Autodesk Inventor part; units mm, degrees
ref_plane "Work Plane1" through (0, 10, 0) normal (0, 1, 0) x (-1, 0, 0)
ref_plane "YZ Plane" through (0, 0, 0) normal (1, 0, 0) x (0, 1, 0)
ref_plane "XY Plane" through (0, 0, 0) normal (0, 0, 1) x (1, 0, 0)
sketch "Sketch1" plane through (0, 0, 0) normal (0, 1, 0) x (-1, 0, 0)
  circle A0 centre (0, 0) radius 50
  dimension "d0" = 100
extrude "Extrusion1" add sketch "Sketch1" along normal blind 20
sketch "Sketch2" plane through (0, 20, 0) normal (0, 1, 0) x (1, 0, 0)
  line L0 (60.9024, 0) -> (39.0976, 0) construction
  circle A0 centre (0, 0) radius 50
  line L1 (60.9024, 10.5) -> (39.0976, 10.5)
  line L2 (39.0976, -10.5) -> (60.9024, -10.5)
  arc A1 (60.9024, -10.5) -> (60.9024, 10.5) centre (60.9024, 0) ccw
  arc A2 (39.0976, 10.5) -> (39.0976, -10.5) centre (39.0976, 0) ccw
  point P0 (50, 0)
  dimension "d3" = 21
extrude "Extrusion2" cut sketch "Sketch2" against normal blind 20 contours A0 L2 A2 L1 | A0 L1 A1 L2 picked at (42.7317, 0)
pattern_circular "Circular Pattern1" count 6 over 360 about axis through (0, -10, 0) along (0, 1, 0) of "Extrusion2"
sketch "Sketch3" plane through (48.8851, 20, 10.5) normal (0, 0, -1) x (-1, 0, 0)
  point P0 (48.8851, -20)
sketch "Sketch4" plane through (0, 20, 0) normal (0, 1, 0) x (1, 0, 0)
  point P0 (0, 0)
ref_plane "Work Plane1" through (0, 10, 0) normal (0, 1, 0) x (-1, 0, 0)
sketch "Sketch5" plane through (0, 10, 0) normal (0, 1, 0) x (-1, 0, 0)
  line L0 (-15.3493, 47.5857) -> (-10.4555, 39.1095)
  arc A0 (-28.6421, 28.6095) -> (-10.4555, 39.1095) centre (-19.5488, 33.8595) ccw
  line L1 (-28.6421, 28.6095) -> (-33.5358, 37.0857)
  arc A1 (-33.5358, 37.0857) -> (-48.8851, 10.5) centre (0, 0) ccw
  line L2 (-48.8851, 10.5) -> (-39.0976, 10.5)
  arc A2 (-39.0976, -10.5) -> (-39.0976, 10.5) centre (-39.0976, 0) ccw
  line L3 (-39.0976, -10.5) -> (-48.8851, -10.5)
  arc A3 (-48.8851, -10.5) -> (-33.5358, -37.0857) centre (0, 0) ccw
  line L4 (-33.5358, -37.0857) -> (-28.6421, -28.6095)
  arc A4 (-10.4555, -39.1095) -> (-28.6421, -28.6095) centre (-19.5488, -33.8595) ccw
  line L5 (-10.4555, -39.1095) -> (-15.3493, -47.5857)
  arc A5 (-15.3493, -47.5857) -> (15.3493, -47.5857) centre (0, 0) ccw
  line L6 (15.3493, -47.5857) -> (10.4555, -39.1095)
  arc A6 (28.6421, -28.6095) -> (10.4555, -39.1095) centre (19.5488, -33.8595) ccw
  line L7 (28.6421, -28.6095) -> (33.5358, -37.0857)
  arc A7 (33.5358, -37.0857) -> (48.8851, -10.5) centre (0, 0) ccw
  line L8 (48.8851, -10.5) -> (39.0976, -10.5)
  arc A8 (39.0976, 10.5) -> (39.0976, -10.5) centre (39.0976, 0) ccw
  line L9 (39.0976, 10.5) -> (48.8851, 10.5)
  arc A9 (48.8851, 10.5) -> (33.5358, 37.0857) centre (0, 0) ccw
  line L10 (33.5358, 37.0857) -> (28.6421, 28.6095)
  arc A10 (10.4555, 39.1095) -> (28.6421, 28.6095) centre (19.5488, 33.8595) ccw
  line L11 (10.4555, 39.1095) -> (15.3493, 47.5857)
  arc A11 (15.3493, 47.5857) -> (-15.3493, 47.5857) centre (0, 0) ccw
  line L12 (15.3493, -47.5857) -> (10.4555, -39.1095)
  line L13 (12.9024, -43.3476) -> (31.0889, -32.8476)
  line L14 (28.6421, -28.6095) -> (33.5358, -37.0857)
  line L15 (43.9913, -10.5) -> (43.9913, 10.5)
  line L16 (31.0889, 32.8476) -> (12.9024, 43.3476)
  line L17 (15.3493, 47.5857) -> (10.4555, 39.1095)
  line L18 (-10.4555, 39.1095) -> (-15.3493, 47.5857)
  line L19 (-12.9024, 43.3476) -> (-31.0889, 32.8476)
  line L20 (-39.0976, 10.5) -> (-48.8851, 10.5)
  line L21 (-43.9913, 10.5) -> (-43.9913, -10.5)
  line L22 (-28.6421, -28.6095) -> (-33.5358, -37.0857)
  line L23 (-31.0889, -32.8476) -> (-12.9024, -43.3476)
  line L24 (-15.3493, -47.5857) -> (-10.4555, -39.1095)
sketch "Sketch6" plane through (-15.3493, 0, 47.5857) normal (-0.866, 0, -0.5) x (-0.5, 0, 0.866)
  point P0 (-48.8851, 0)
sketch "Sketch7" plane through (15.3493, 0, 47.5857) normal (0.866, 0, -0.5) x (-0.5, 0, -0.866)
  line L0 (0, 10) -> (9.7874, 10)
  circle A0 centre (4.8937, 10) radius 1
  point P0 (48.8851, 0)
  dimension "d10" = 2
sweep "Sweep1" add profiles "Sketch7" path "Sketch5" path curves L19
pattern_circular "Circular Pattern2" count 6 over 360 about axis through (0, -10, 0) along (0, 1, 0) of "Sweep1"
sketch "Sketch8" plane through (0, 0, 0) normal (0, -1, 0) x (1, 0, 0)
  circle A0 centre (0, 0) radius 15
  dimension "d16" = 30
extrude "Extrusion3" cut sketch "Sketch8" against normal up to next
properties part number "Holder"
The model under review builds one solid part; all positions refer to its coordinate system, in mm. Coordinates: 2 decimals unless noted, no trailing zeros. Write each loop counter-clockwise with the first axis right and the second up, starting at its lowest first coordinate (ties: lowest second). Pieces come first, ordered by that corner, then holes. Notation, with made-up numbers: (21.25, -37) -> (76.25, -37) arc R27 cw to (76.25, -20) -> close; hole circle Ø6 at (-33.5, 55). An arc over 180 degrees is marked (long way). Answer in a Markdown table with one row per item.
1. Clearance check with flat-ended pins moving along their axes: pin 1 Ø1.5 at (x, z) = (-0.5, 40) entering from -Y; pin 2 Ø8 at (x, y) = (42.5, 5) entering from -Z; pin 3 Ø8 at (x, y) = (22, 9.5) entering from -Z; pin 4 Ø5 at (x, y) = (-43.5, 14) entering from +Z. State where each tip first meets the part, or that it passes through.
Answers below:
| item | result |
|---|---|
| pin 1 | stops at y = 0 |
| pin 2 | stops at z = -31.9 |
| pin 3 | stops at z = -41.54 |
| pin 4 | stops at z = 28.62 |
2. We need section D-D, the plane x = -41. State the section outline as (y, z) points.
Answers below:
| item | result |
|---|---|
| outline | (0, -28.62) -> (20, -28.62) -> (20, -10.5) -> (0, -10.5) -> close; (0, 10.5) -> (20, 10.5) -> (20, 28.62) -> (0, 28.62) -> close |
3. Draft analysis for pull direction X (two halves, no side actions). For faces 1 (the flat face through (-30.511, 10.14, 31.846)), 2 (the cylindrical face through (-43.19, 9.86, 25.19)), 3 (the cylindrical face through (-14.5, 10.14, -24.653)), 4 (the flat face through (12, 20, 12)), state which applies: +X half, -X half, draft (parallel to the pull), parting line (faces both ways), or undercut.
Answers below:
| item | result |
|---|---|
| face 1 | undercut |
| face 2 | -X half |
| face 3 | undercut |
| face 4 | draft |
4. We need section C-C, the plane z = 0. Give the number of separate pieces and of enclosed holes in the cut face, and give its area (3 significant figures).
Answers below:
| item | result |
|---|---|
| separate pieces | 4 |
| enclosed holes | 0 |
| area | 550 mm^2 |
5. Wall thickness on probe 1 along Z at (x, y) = (0, 12.25); probe 2 along Z at (x, y) = (40.5, 15.5); probe 3 along X at (y, z) = (17.5, -7): over which ranges is each line inside the solid? List them lowest first. Write a range as [from, to].
Answers below:
| item | result |
|---|---|
| probe 1 | z = [-50, -15], [15, 50] |
| probe 2 | z = [-29.32, -10.5], [10.5, 29.32] |
| probe 3 | x = [-31.27, -13.27], [13.27, 31.27] |
6. We need section A-A, the plane x = 0. State the section outline as (y, z) points.
Answers below:
| item | result |
|---|---|
| outline | (0, -50) -> (20, -50) -> (20, -15) -> (0, -15) -> close; (0, 15) -> (20, 15) -> (20, 50) -> (0, 50) -> close |
